Study the drawing (mm; zero at the part's minimum x, y, z) and answer. Round coordinates to 2 decimals unless told otherwise and drop trailing zeros. Write each loop counter-clockwise with the first axis right and the second up, starting at its lowest first coordinate (ties: lowest second). Pieces come first, ordered by that corner, then holes. Notation, with made-up numbers: (18.5, 5) -> (22.5, 5) arc R33 cw to (22.5, 39) -> close; hole circle Ø10 at (84, 72). An arc over 180 degrees is marked (long way). Return JSON: item names as keys, results as strings.
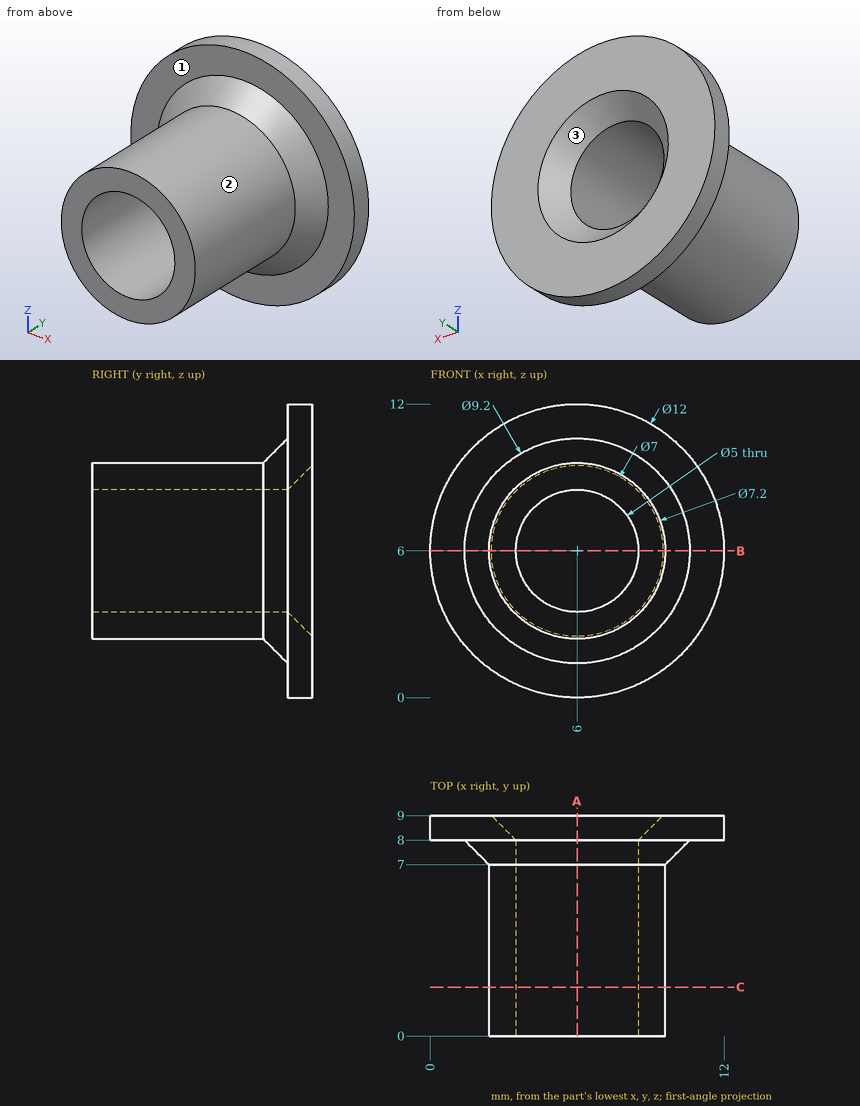
Item 1: Section C-C (y = 2) is taken. Give the vertices of the cut face in (x, z), then the cut area to 3 significant figures.
Worked answers:
{"outline": "circle Ø7.2 at (6, 6); hole circle Ø5 at (6, 6)", "area": "21.1 mm2"}
Item 2: Section A-A (x = 6) is taken. Give the vertices of the cut face in (y, z).
Worked answers:
{"outline": "(0, 2.4) -> (7, 2.4) -> (8, 1.4) -> (8, 0) -> (9, 0) -> (9, 2.5) -> (8, 3.5) -> (0, 3.5) -> close; (0, 8.5) -> (8, 8.5) -> (9, 9.5) -> (9, 12) -> (8, 12) -> (8, 10.6) -> (7, 9.6) -> (0, 9.6) -> close"}
Item 3: For a pull along Z with two mould halves and no side action, classify the marked faces 1, 2 and 3 as released by +Z, released by -Z, zero draft, split by the parting line, or undercut.
Worked answers:
{"face 1": "zero draft", "face 2": "split by the parting line", "face 3": "undercut"}
Item 4: Straight lines are drawn through the part: L1, parallel to Z at x = 6, y = 5; L2, parallel to Y at x = 9.5, z = 10. For each, find the intervals that lie inside material, in ascending order. Write a range as [from, to].
Worked answers:
{"L1": "z = [2.4, 3.5], [8.5, 9.6]", "L2": "y = [8, 9]"}
Item 5: Section B-B (z = 6) is taken. Give the vertices of the cut face in (x, y), then the cut area to 3 significant figures.
Worked answers:
{"outline": "(0, 8) -> (1.4, 8) -> (2.4, 7) -> (2.4, 0) -> (3.5, 0) -> (3.5, 8) -> (2.5, 9) -> (0, 9) -> close; (8.5, 0) -> (9.6, 0) -> (9.6, 7) -> (10.6, 8) -> (12, 8) -> (12, 9) -> (9.5, 9) -> (8.5, 8) -> close", "area": "24.6 mm2"}
Item 6: Flat-ended cylindrical pins translate along their axes: pin 1 (1 mm diameter, centred on x = 3.5, y = 3.5, fed in from +Z); pin 2 (6.5 mm diameter, centred on x = 6, z = 6, fed in from +Y); pin 3 (5 mm diameter, centred on y = 4, z = 5, fed in from -X). Find the tip coordinate at first contact, or state that the pin passes through.
Worked answers:
{"pin 1": "stops at z = 8.99", "pin 2": "stops at y = 8.75", "pin 3": "stops at x = 2.4"}
